Input: part model. Units: mm. Frame: model coordinates. A direction names the side the tool comes from. Coordinates: 2 decimals unless noted, no trailing zeros. Loops run counter-clockwise (first coordinate to the right, second up) from the corner with the lowest first, then second, coordinate; pieces in that order, holes last. Notation, with made-up numbers: (42, 52) -> (88, 52) arc R33 cw to (88, 86) -> close; hole circle Ø3 at (76, 10.5). An arc over 180 degrees is marked (long way). Put each result on its own line as item: value. Start each with the question number.
1) Material intervals for L1, parallel to Y at x = 33, z = -5; L2, parallel to Z at x = -8.5, y = 50; L3, parallel to Z at x = -6.5, y = 50, sorted ascending.
2) Contact query for flat-ended pins moving along their axis: P1, Ø3, axis at x = -4.5, z = 11, coming from the +Y side; P2, Ø5, axis at y = 74.5, z = 23.5, coming from the +X side; P3, Ø5, axis at y = 53, z = 20.5, coming from the +X side. Output: stop coordinate, or through.
3) Cut plane B-B (y = 19). Return the cut outline in (x, z), plus the area to 3 significant figures.
4) Pull-direction query (Z, two-part tool) for faces 1 (the flat face through (10.645, 19.697, 29.077)), 2 (the flat face through (1, 0, 1)), 3 (the conical face through (-6.429, 25.235, 48.965)); classes: pulls with the +Z half, pulls with the -Z half, needs draft (parallel to the pull), parting line crosses it, or undercut.
5) Cut plane A-A (y = 56). Return the cut outline in (x, z).
6) Set-up query: faces 4 (the cylindrical face through (9.92, 30.57, 24.58)), 5 (the flat face through (20.9, 19.4, 0.4)), 6 (the flat face through (-33, 12, 1)). Return all of +Z, -Z, +X, -X, +Y, -Y with unobstructed straight access to the full face (end or side cutting, diameter ignored); none if empty.
from build123d import *

# Parameters (mm, degrees)
CUT_EXTRUDE1_DEPTH      = 116.217186218
CUT_EXTRUDE4_DEPTH      = 116.217186218
CUT_EXTRUDE4_DEPTH_BACK = 36
SKETCH7_R               = 21
SKETCH7_10_R            = 21
CUT_EXTRUDE7_DEPTH      = 116.217186218


with BuildPart() as part:
    # Sketch2 → Revolve3 (revolve)
    with BuildSketch(Plane.XY, mode=Mode.PRIVATE) as revolve3_sk:
        with BuildLine():
            Line((0, 0), (-55, 0))
            Line((-55, 0), (-43.925913783, 49.773131451))
            ThreePointArc((-43.925913783, 49.773131451), (-28.153233249, 75.10549042), (0, 85))
            Line((0, 85), (0, 0))
        make_face()
    revolve(revolve3_sk.sketch.rotate(Axis((0, 85, 0), (0, -1, 0)), 180), axis=Axis((0, 85, 0), (0, -1, 0)))

    # Sketch6 → Cut-Extrude1 (cut, symmetric)
    with BuildSketch(Plane.XY):
        with BuildLine():
            Line((-321.935585995, 12), (-52.330105004, 12))
            Line((-52.330105004, 12), (-23.212875062, 12))
            Line((-23.212875062, 12), (-15, 82.426406871))
            ThreePointArc((-15, 82.426406871), (0, 85), (15, 82.426406871))
            Line((15, 82.426406871), (21.593288149, 12))
            Line((21.593288149, 12), (52.330105004, 12))
            Line((52.330105004, 12), (321.935585995, 12))
            Line((321.935585995, 12), (321.935585995, 551.210961982))
            Line((321.935585995, 551.210961982), (-321.935585995, 551.210961982))
            Line((-321.935585995, 551.210961982), (-321.935585995, 12))
        make_face()
    cut_extrude1 = extrude(amount=CUT_EXTRUDE1_DEPTH, both=True, mode=Mode.SUBTRACT)

    # Sketch7 → Cut-Extrude4 (cut, two sides: drawn at the far end of the back side and taken through both)
    with BuildSketch(Plane(origin=(0, 0, 0), x_dir=(0, 0, -1), z_dir=(1, 0, 0)).offset(-CUT_EXTRUDE4_DEPTH_BACK)):
        with Locations(Location((0, 50, 0), (0, 0, 270))):
            Circle(SKETCH7_R)
    extrude(amount=CUT_EXTRUDE4_DEPTH + CUT_EXTRUDE4_DEPTH_BACK, mode=Mode.SUBTRACT)

    # Sketch7_10 → Cut-Extrude7 (cut, through all)
    with BuildSketch(Plane(origin=(0, 0, 0), x_dir=(0, 0, -1), z_dir=(1, 0, 0))):
        with BuildLine():
            Line((30.789792632, 12), (44.134487224, 12))
            Line((44.134487224, 12), (36.116862443, 48.03568586))
            ThreePointArc((36.116862443, 48.03568586), (0, 77), (-36.116862443, 48.03568586))
            Line((-36.116862443, 48.03568586), (-44.134487224, 12))
            Line((-44.134487224, 12), (-30.789792632, 12))
            Line((-30.789792632, 12), (-27.316320114, 27.61172641))
            ThreePointArc((-27.316320114, 27.61172641), (-24.523281701, 30.585476266), (-20.574001178, 29.562033479))
            ThreePointArc((-20.574001178, 29.562033479), (0, 21), (20.574001178, 29.562033479))
            ThreePointArc((20.574001178, 29.562033479), (24.523281701, 30.585476266), (27.316320114, 27.61172641))
            Line((27.316320114, 27.61172641), (30.789792632, 12))
        make_face()
        with Locations((0, 50)):
            Circle(SKETCH7_10_R, mode=Mode.SUBTRACT)
    extrude(amount=CUT_EXTRUDE7_DEPTH, mode=Mode.SUBTRACT)

    # Mirror1: Cut-Extrude1 across plane
    add(cut_extrude1.mirror(Plane(origin=(0, 0, 0), x_dir=(0, 0, 1), z_dir=(1, 0, 0))), mode=Mode.SUBTRACT)


solid = part.part
Results found:
1. L1: y = 0 to 12
1. L2: z = -43.04 to -21, 21 to 43.04
1. L3: z = -43.39 to -21, 21 to 43.39
2. P1: stops at y = 83.79
2. P2: stops at x = 15.98
2. P3: stops at x = 0
3. outline: (-20.94, -46.25) arc R50.77 ccw to (20.94, -46.25) -> (20.94, -42.58) -> (0, -42.58) -> (0, -29.23) -> (20.94, -29.23) -> (20.94, 29.23) -> (0, 29.23) -> (0, 42.58) -> (20.94, 42.58) -> (20.94, 46.25) arc R50.77 ccw to (-20.94, 46.25) -> close
3. area: 3,570 mm2
4. face 1: undercut
4. face 2: needs draft
4. face 3: parting line crosses it
5. outline: (-17.47, -38.26) arc R42.06 ccw to (17.47, -38.26) -> (17.47, -33.36) -> (0, -33.36) -> (0, -20.12) -> (-17.47, -20.12) -> close; (-17.47, 20.12) -> (0, 20.12) -> (0, 33.36) -> (17.47, 33.36) -> (17.47, 38.26) arc R42.06 ccw to (-17.47, 38.26) -> close
6. face 4: +X
6. face 5: +Z, -Z, +X, +Y
6. face 6: +Z, -Z, -X, +Y
